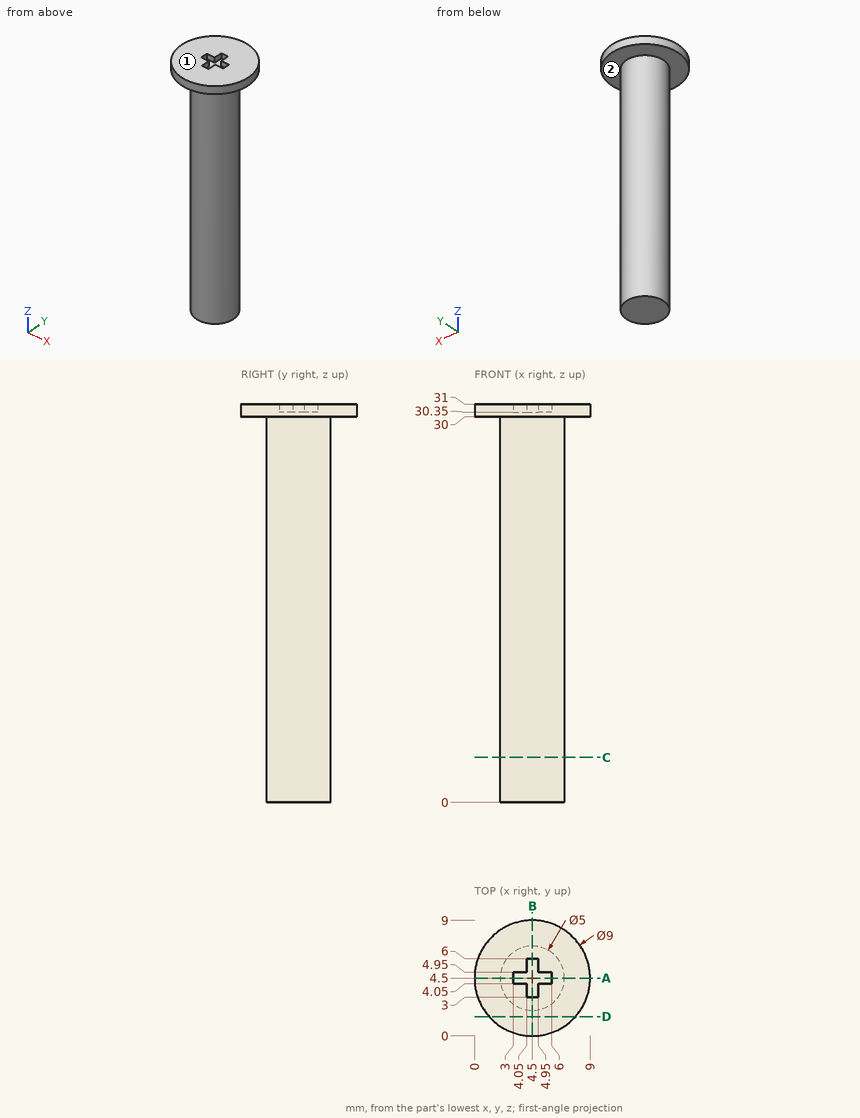
Could you check a few things on this drawing? It's one solid part, dimensions in mm from its lowest x, y, z. A direction names the side the tool comes from. Give positions to 0.01 mm unless a question says otherwise; leave off trailing zeros. Write each loop counter-clockwise with the first axis right and the second up, starting at its lowest first coordinate (ties: lowest second). Pieces come first, ordered by that corner, then holes. Notation, with made-up numbers: (-26, -14.75) - (6, -14.75) arc R20 cw to (6, 15.25) - close; hole circle Ø4 at (78.5, 9). An arc over 180 degrees is marked (long way). Use CSV: the item, a comma, the result in double quotes. Start each with the question number.
Item 1: I want a section at C-C, the plane z = 3.5. Please give me the cut outline in (x, y).
Item 2: For the marked faces 1 and 2, which set-ups out of +Z, -Z, +X, -X, +Y, -Y let a thin tool reach every point of the face, with its end or its side?
Item 3: If I drill on line 1 along Z through (x, y) = (5.5, 8); line 2 along X through (y, z) = (2.25, 26.5); line 3 along Y through (x, z) = (5.5, 4), over which ranges is the centre line in solid material (lowest first)?
Item 4: I'm going to push flat-ended pins straight in: pin 1 (2 mm diameter, centred on x = 3.5, z = 24.5, fed in from -Y); pin 2 (1.5 mm diameter, centred on x = 4, y = 4.5, fed in from +Z); pin 3 (2 mm diameter, centred on x = 5, z = 22.5, fed in from +Y); pin 4 (0.7 mm diameter, centred on x = 5.5, z = 30.5, fed in from -Y). Where does each tip first touch, or does it pass through?
Item 5: I want a section at D-D, the plane y = 1.5. Please give me the cut outline in (x, z), then the cut area to 3 significant figures.
Item 6: I want a section at A-A, the plane y = 4.5. Please give me the cut outline in (x, z).
Findings:
1,outline,"circle Ø5 at (4.5, 4.5)"
2,face 1,"+Z, +X, -X, +Y, -Y"
2,face 2,"-Z"
3,line 1,"z = 30 to 31"
3,line 2,"x = 3.41 to 5.59"
3,line 3,"y = 2.21 to 6.79"
4,pin 1,"stops at y = 2"
4,pin 2,"stops at z = 31"
4,pin 3,"stops at y = 7"
4,pin 4,"stops at y = 0.05"
5,outline,"(1.15, 30) - (7.85, 30) - (7.85, 31) - (1.15, 31) - close"
5,area,"6.71 mm2"
6,outline,"(0, 30) - (2, 30) - (2, 0) - (7, 0) - (7, 30) - (9, 30) - (9, 31) - (6, 31) - (6, 30.35) - (3, 30.35) - (3, 31) - (0, 31) - close"
